```python
from build123d import *

# Parameters (mm, degrees)
BOSS_EXTRUDE1_DEPTH = 127
SKETCH2_R           = 10.16
CUT_EXTRUDE1_DEPTH  = 157.585578439
CHAMFER1_SIZE       = 5.08
SKETCH3_W           = 19.05
SKETCH3_H           = 76.2
CUT_EXTRUDE2_DEPTH  = 12.7
FILLET1_R           = 12.7
CUT_EXTRUDE4_DEPTH  = 31.762338
FILLET2_R           = 12.7
FILLET3_R           = 12.7
FILLET4_R           = 12.7
FILLET5_R           = 12.7


with BuildPart() as part:
    # Sketch1 → Boss-Extrude1 (new body)
    with BuildSketch(Plane.XY):
        Polygon((0, 0), (0.954886233, 50.8), (39.054886233, 50.083835325), (76.2, 17.617670651), (76.2, -1.432329349), align=None)
    extrude(amount=BOSS_EXTRUDE1_DEPTH)

    # Sketch2 → Cut-Extrude1 (cut, through all)
    with BuildSketch(Plane(origin=(0.954886233, 50.8, 0), x_dir=(0.9998233837023289, -0.01879365323787949, 0), z_dir=(0.01879365323787949, 0.999823383702329, 0))):
        with Locations(Location((19.05, -25.4, 0), (0, 0, 180))):
            Circle(SKETCH2_R)
    extrude(amount=-CUT_EXTRUDE1_DEPTH, mode=Mode.SUBTRACT)

    # Chamfer1
    chamfer1_edges = [part.edges().sort_by_distance(p)[0] for p in [
        (30.159727271, 50.251037389, 25.4),
    ]]
    chamfer(chamfer1_edges, length=CHAMFER1_SIZE)

    # Sketch3 → Cut-Extrude2 (cut)
    with BuildSketch(Plane(origin=(0.954886233, 50.8, 0), x_dir=(0.9998233837023289, -0.01879365323787949, 0), z_dir=(0.01879365323787949, 0.999823383702329, 0))):
        with Locations((9.525, -88.9)):
            Rectangle(SKETCH3_W, SKETCH3_H)
    extrude(amount=-CUT_EXTRUDE2_DEPTH, mode=Mode.SUBTRACT)

    # Fillet1
    fillet1_edges = [part.edges().sort_by_distance(p)[0] for p in [
        (19.882181994, 44.093102419, 50.8),
    ]]
    fillet(fillet1_edges, radius=FILLET1_R)

    # Sketch10 → Cut-Extrude4 (cut)
    with BuildSketch(Plane(origin=(0.954886233, 50.8, 0), x_dir=(0.9998233837023289, -0.01879365323787949, 0), z_dir=(0.01879365323787949, 0.999823383702329, 0))):
        with BuildLine():
            Line((75.755441679, -50.8), (59.753441679, -50.8))
            ThreePointArc((59.753441679, -50.8), (47.053441679, -63.5), (59.753441679, -76.2))
            Line((59.753441679, -76.2), (75.755441679, -76.2))
            Line((75.755441679, -76.2), (75.755441679, -50.8))
        make_face()
    extrude(amount=-CUT_EXTRUDE4_DEPTH, mode=Mode.SUBTRACT)

    # Fillet2
    fillet2_edges = [part.edges().sort_by_distance(p)[0] for p in [
        (76.2, 8.092670651, 127),
    ]]
    fillet(fillet2_edges, radius=FILLET2_R)

    # Fillet3
    fillet3_edges = [part.edges().sort_by_distance(p)[0] for p in [
        (0.358103418, 19.051121513, 127),
    ]]
    fillet(fillet3_edges, radius=FILLET3_R)

    # Fillet4
    fillet4_edges = [part.edges().sort_by_distance(p)[0] for p in [
        (0.477443116, 25.4, 0),
    ]]
    fillet(fillet4_edges, radius=FILLET4_R)

    # Fillet5
    fillet5_edges = [part.edges().sort_by_distance(p)[0] for p in [
        (76.2, 8.092670651, 0),
    ]]
    fillet(fillet5_edges, radius=FILLET5_R)


solid = part.part
```
Design review of the part built by this model. Coordinates are the model's own, in mm. A direction names the side the tool comes from. Coordinates: 2 decimals unless noted, no trailing zeros. Order: outer loops, then holes, each group sorted by start corner. A loop starts at its lowest first (then second) coordinate and runs counter-clockwise, first axis right, second up.
1) Take a section at B-B, the plane x = 65. Give the boundary of the cut face in (y, z).
2) For faces 1 (the cylindrical face through (4.105, 25.688, 3.819)), 2 (the flat face through (4, 44, 50.8)), 3 (the flat face through (38, 19, 127)), 4 (the cylindrical face through (47.586, 27.751, 63.221)), 5 (the cylindrical face through (20.805, 22.798, 35.474)), list the 3-axis set-ups (+Z, -Z, +X, -X, +Y, -Y) from which the entire face can be reached by the end or side of a thin tool; tool diameter is ignored.
3) Clearance check with flat-ended pins moving along their axes: pin 1 (2 mm diameter, centred on x = 3.5, y = 47.5, fed in from +Z); pin 2 (8 mm diameter, centred on x = 25.5, z = 114, fed in from -Y); pin 3 (8 mm diameter, centred on x = 48, z = 85.5, fed in from -Y). State where each tip first meets the part, or that it passes through.
4) Take a section at C-C, the plane z = 70. Give the boundary of the cut face in (x, y), and give its area (3 significant figures).
5) Take a section at A-A, the plane z = 107.5. Give the boundary of the cut face in (x, y).
6) Mouldability with a two-part tool opening along Z and no side actions: class faces 6 (the flat face through (57.367, 34.078, 76.722)), 7 (the flat face through (65, 22, 50.8)), 8 (the cylindrical face through (4.2, 19.2, 123.4)), 9 (the flat face through (66, 23, 76.2)) as +Z half, -Z half, draft (parallel to the pull), parting line (faces both ways), or undercut.
7) Take a section at D-D, the plane x = 44. Give the boundary of the cut face in (y, z), and give its area (3 significant figures).
8) Wall thickness on line 1 along Y through (x, z) = (63.5, 10.5); line 2 along Z through (x, y) = (28.5, 22.5); line 3 along X through (y, z) = (31, 22): over which ranges is each line inside the solid? List them lowest first.
Returned:
1. outline: (-1.22, 0.09) - (27.41, 0.09) - (27.41, 50.8) - (17.83, 50.8) - (17.83, 76.2) - (27.41, 76.2) - (27.41, 126.91) - (-1.22, 126.91) - close
2. face 1: -Z, -X, +Y
2. face 2: +Z, -X, +Y
2. face 3: +Z, +X, -X, +Y, -Y
2. face 4: +X
2. face 5: none
3. pin 1: stops at z = 50.8
3. pin 2: stops at y = -0.55
3. pin 3: stops at y = -0.98
4. outline: (0, 0) - (76.2, -1.43) - (76.2, 17.62) - (76.1, 17.7) - (76.1, 17.62) - (49.19, 18.13) - (49.62, 40.85) - (39.05, 50.08) - (20, 50.44) - (19.76, 37.74) - (0.72, 38.1) - close
4. area: 2,710 mm2
5. outline: (0, 0) - (76.2, -1.43) - (76.2, 17.62) - (39.05, 50.08) - (20, 50.44) - (19.76, 37.74) - (0.72, 38.1) - close
6. face 6: draft
6. face 7: undercut
6. face 8: +Z half
6. face 9: undercut
7. outline: (-0.83, 0) - (45.76, 0) - (45.76, 127) - (-0.83, 127) - close
7. area: 5,920 mm2
8. line 1: y = -1.19 to 28.72
8. line 2: z = 0 to 20.73, 30.07 to 127
8. line 3: x = 0.58 to 10.06, 29.21 to 60.89
